The listing builds one solid part. Answer for the finished solid, in the listing's coordinates (mm). Face numbers are marked on the shaded views. A direction names the side the tool comes from. Round coordinates to 2 decimals unless told otherwise and drop trailing zeros. Loops run counter-clockwise (first coordinate to the right, second up) from the corner with the lowest first, then second, coordinate; pieces in that order, holes last. Notation, with made-up numbers: (64.5, 24) -> (100.5, 24) arc R24 ccw to (100.5, 52) -> close; hole circle Ø5 at (89.5, -24). An arc over 180 degrees is marked (long way). One line per question, with ' | ' between items.
from build123d import *

# Parameters (mm, degrees)
SKETCH2_OUTSIDE_W  = 39.511
SKETCH2_OUTSIDE_H  = 39.51
SKETCH2_OUTSIDE_R  = 2.413
CUT_EXTRUDE1_DEPTH = 2.38125
FILLET1_R          = 2.54
FILLET2_R          = 0.79375


with BuildPart() as part:
    # Sketch1 → Revolve1 (revolve)
    with BuildSketch(Plane.XY):
        with BuildLine():
            Line((-5.55625, 0), (-14.2875, 0))
            Line((-14.2875, 0), (-14.2875, -2.38125))
            Line((-14.2875, -2.38125), (-2.38125, -2.38125))
            Line((-2.38125, -2.38125), (-2.38125, 0))
            ThreePointArc((-2.38125, 0), (-3.359821243, 8.138211612), (-6.239746425, 15.812462121))
            ThreePointArc((-6.239746425, 15.812462121), (-8.380030966, 16.49032242), (-9.057891265, 14.350037879))
            ThreePointArc((-9.057891265, 14.350037879), (-6.444317544, 7.385544643), (-5.55625, 0))
        make_face()
    revolve(axis=Axis((0, -2.38125, 0), (0, 1, 0)))

    # Sketch2 outside → Cut-Extrude1 (cut)
    with BuildSketch(Plane.XZ.offset(2.38125)):
        with Locations((0.0005, 0)):
            Rectangle(SKETCH2_OUTSIDE_W, SKETCH2_OUTSIDE_H)
        with BuildLine():
            Line((-10.4775, 3.81), (-6.963318623, 3.81))
            ThreePointArc((-6.963318623, 3.81), (0, 7.9375), (6.963318623, 3.81))
            Line((6.963318623, 3.81), (10.4775, 3.81))
            ThreePointArc((10.4775, 3.81), (14.2875, 0), (10.4775, -3.81))
            Line((10.4775, -3.81), (6.963318623, -3.81))
            ThreePointArc((6.963318623, -3.81), (0, -7.9375), (-6.963318623, -3.81))
            Line((-6.963318623, -3.81), (-10.4775, -3.81))
            ThreePointArc((-10.4775, -3.81), (-14.2875, 0), (-10.4775, 3.81))
        make_face(mode=Mode.SUBTRACT)
        with Locations((-10.4775, 0)):
            Circle(SKETCH2_OUTSIDE_R)
        with Locations((10.4775, 0)):
            Circle(SKETCH2_OUTSIDE_R)
    extrude(amount=-CUT_EXTRUDE1_DEPTH, mode=Mode.SUBTRACT)

    # Fillet1
    fillet1_edges = [part.edges().sort_by_distance(p)[0] for p in [
        (-6.963318623, -1.190625, -3.81),
        (6.963318623, -1.190625, -3.81),
        (6.963318623, -1.190625, 3.81),
        (-6.963318623, -1.190625, 3.81),
    ]]
    fillet(fillet1_edges, radius=FILLET1_R)

    # Fillet2
    fillet2_edges = [part.edges().sort_by_distance(p)[0] for p in [
        (5.55625, 0, 0),
    ]]
    fillet(fillet2_edges, radius=FILLET2_R)


solid = part.part
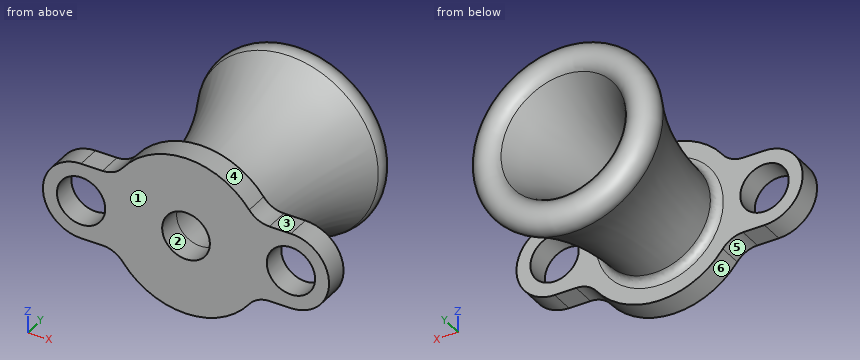
Q1. A cutting plane is placed at C-C on z = 0. Give the number of separate pieces and of enclosed holes in the cut face, plus the area to 3 significant figures.
Numbers:
separate pieces: 4 | enclosed holes: 0 | area: 141 mm^2
Q2. For a pull along Z with two mould halves and no side action, classify the marked faces 1, 2 and 3 as pulls with the +Z half, pulls with the -Z half, needs draft (parallel to the pull), parting line crosses it, or undercut.
Numbers:
face 1: needs draft | face 2: undercut | face 3: pulls with the +Z half
Q3. For the marked faces 4, 5 and 6, determine the directions among +Z, -Z, +X, -X, +Y, -Y from which every point of the face is accessible in a straight line to the end or side of a thin tool.
Numbers:
face 4: +Z, -Y | face 5: -Z, -X, -Y | face 6: -Z, -Y
Q4. A cutting plane is placed at A-A on x = 9.75. Give the vertices of the cut face in (y, z).
Numbers:
outline: (-2.38, -3.81) -> (0, -3.81) -> (0, -2.3) -> (-2.38, -2.3) -> close; (-2.38, 2.3) -> (0, 2.3) -> (0, 3.81) -> (-2.38, 3.81) -> close
Q5. Given pin 1 Ø2.5 at (x, y) = (9.5, -1.5) entering from -Z; pin 2 Ø4 at (x, z) = (0.5, -3) entering from +Y; pin 3 Ø2.5 at (x, y) = (9.5, -1.5) entering from +Z; pin 4 Ø5.5 at (x, z) = (10.48, 0) entering from -Y, each flat-ended and moving along its own axis, determine where each tip first touches the part or whether it passes through.
Numbers:
pin 1: z = -3.81 | pin 2: y = 13.25 | pin 3: z = 3.81 | pin 4: y = -2.38
Q6. A cutting plane is placed at B-B on y = 6.5. Give the vertices of the cut face in (x, z).
Numbers:
outline: circle Ø12.48 at (0, 0); hole circle Ø6 at (0, 0)
Q7. Find the intervals of material crossed by line 1 (Y direction, x = 11.5, z = -2.75); line 2 (Z direction, x = 12, y = -0.5); line 3 (Z direction, x = -2, y = 5), in increasing order. Write a range as from..to.
Numbers:
line 1: -2.38..0 | line 2: -3.49..-1.87, 1.87..3.49 | line 3: -5.61..-1.88, 1.88..5.61
